Work out the finished part from the listing and answer in its coordinate system (mm). Round coordinates to 2 decimals unless told otherwise and drop trailing zeros. Loops run counter-clockwise (first coordinate to the right, second up) from the corner with the lowest first, then second, coordinate; pieces in that order, holes last. Notation, with made-up numbers: (69.5, 12) -> (105.5, 12) arc R11 cw to (105.5, 31) -> close; hole circle Ø9 at (-4, 13). An arc over 180 degrees is marked (long way). Use one line per item in the form item = value.
```python
from build123d import *

# Parameters (mm, degrees)
SKETCH_1_R               = 57.5
SKETCH_1_R_2             = 45
SKETCH_1_R_3             = 2.5
EXTRUDE_1_DEPTH          = 8.5
PATTERN_CIRCULAR_1_COUNT = 4


with BuildPart() as part:
    # Sketch 1 → Extrude 1 (new body)
    with BuildSketch(Plane(origin=(0, 0, 0), x_dir=(1, 0, 0), z_dir=(0, 1, 0))):
        with Locations(Location((0, 0, 0), (0, 0, 270))):
            Circle(SKETCH_1_R)
        with Locations(Location((0, 0, 0), (0, 0, 270))):
            Circle(SKETCH_1_R_2, mode=Mode.SUBTRACT)
        with Locations(Location((0, 50.5, 0), (0, 0, 270))):
            Circle(SKETCH_1_R_3, mode=Mode.SUBTRACT)
        with Locations(Location((50.5, 0, 0), (0, 0, 270))):
            Circle(SKETCH_1_R_3, mode=Mode.SUBTRACT)
        with Locations(Location((0, -50.5, 0), (0, 0, 270))):
            Circle(SKETCH_1_R_3, mode=Mode.SUBTRACT)
        with Locations(Location((-50.5, 0, 0), (0, 0, 270))):
            Circle(SKETCH_1_R_3, mode=Mode.SUBTRACT)
    extrude(amount=-EXTRUDE_1_DEPTH)

    # Sketch 2 → Cut-Revolve 1 (revolve, cut)
    with BuildSketch(Plane.XY.offset(-50.5), mode=Mode.PRIVATE) as cut_revolve_1_sk:
        Polygon((0, 0), (4.9, 0), (1.6, -3.3), (0, -3.3), align=None)
    cut_revolve_1 = revolve(cut_revolve_1_sk.sketch.rotate(Axis((0, -3.3, -50.5), (0, 1, 0)), 270), axis=Axis((0, -3.3, -50.5), (0, 1, 0)), mode=Mode.SUBTRACT)

    # Pattern Circular 1: Cut-Revolve 1 ×4 about axis
    pattern_circular_1_axis = Axis((0, 0, 0), (0, 1, 0))
    for i in range(1, PATTERN_CIRCULAR_1_COUNT):
        add(cut_revolve_1.rotate(pattern_circular_1_axis, i * 360 / PATTERN_CIRCULAR_1_COUNT), mode=Mode.SUBTRACT)


solid = part.part
```
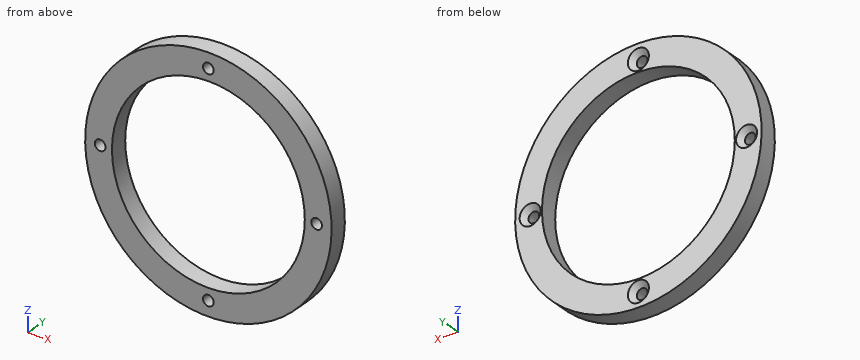
(1) Find section B-B, the plane x = 0. Write down the section's boundary in (y, z).
Completed:
outline = (-8.5, -57.5) -> (0, -57.5) -> (0, -55.4) -> (-2.4, -53) -> (-8.5, -53) -> close; (-8.5, -48) -> (-2.4, -48) -> (0, -45.6) -> (0, -45) -> (-8.5, -45) -> close; (-8.5, 45) -> (0, 45) -> (0, 45.6) -> (-2.4, 48) -> (-8.5, 48) -> close; (-8.5, 53) -> (-2.4, 53) -> (0, 55.4) -> (0, 57.5) -> (-8.5, 57.5) -> close
(2) Find section D-D, the plane z = 50.5. Write down the section's boundary in (x, y).
Completed:
outline = (-27.5, -8.5) -> (-2.5, -8.5) -> (-2.5, -2.4) -> (-4.9, 0) -> (-27.5, 0) -> close; (2.5, -8.5) -> (27.5, -8.5) -> (27.5, 0) -> (4.9, 0) -> (2.5, -2.4) -> close
(3) Find section C-C, the plane x = 50.5. Write down the section's boundary in (y, z).
Completed:
outline = (-8.5, -27.5) -> (0, -27.5) -> (0, -4.9) -> (-2.4, -2.5) -> (-8.5, -2.5) -> close; (-8.5, 2.5) -> (-2.4, 2.5) -> (0, 4.9) -> (0, 27.5) -> (-8.5, 27.5) -> close
(4) Given P1, Ø6.5, axis at x = 0, z = 50.5, coming from the +Y side; P2, Ø5, axis at x = -35.5, y = -4, coming from the +Z side; P3, Ø1.5, axis at y = -1.5, z = -26.5, coming from the +X side; P4, Ø3, axis at x = 30, z = -34, coming from the +Y side, each flat-ended and moving along its own axis, determine where each tip first touches the part or whether it passes through.
Completed:
P1 = -1.65
P2 = 47.09
P3 = 51.41
P4 = 0
(5) Consider L1, parallel to X at y = -5.25, z = 0; L2, parallel to X at y = -6, z = 50.5; L3, parallel to Z at x = 25.5, y = -5.75. Determine where each line is inside the solid, lowest interval first.
Completed:
L1 = -57.5 to -53, -48 to -45, 45 to 48, 53 to 57.5
L2 = -27.5 to -2.5, 2.5 to 27.5
L3 = -51.54 to -37.08, 37.08 to 51.54
(6) Find section A-A, the plane z = 0. Write down the section's boundary in (x, y), then the cut area to 3 significant figures.
Completed:
outline = (-57.5, -8.5) -> (-53, -8.5) -> (-53, -2.4) -> (-55.4, 0) -> (-57.5, 0) -> close; (-48, -8.5) -> (-45, -8.5) -> (-45, 0) -> (-45.6, 0) -> (-48, -2.4) -> close; (45, -8.5) -> (48, -8.5) -> (48, -2.4) -> (45.6, 0) -> (45, 0) -> close; (53, -8.5) -> (57.5, -8.5) -> (57.5, 0) -> (55.4, 0) -> (53, -2.4) -> close
area = 116 mm2
